The listing builds one solid part. Answer for the finished solid, in the listing's coordinates (mm). Round coordinates to 2 decimals unless told otherwise and drop trailing zeros. Write each loop counter-clockwise with the first axis right and the second up, starting at its lowest first coordinate (ties: lowest second). Pieces come first, ordered by that corner, then holes. Notation, with made-up numbers: M 16,-7.5 L 26,-7.5 A25 ccw 26,7.5 Z; hole C 36.5,72.5 d11. An arc over 180 degrees is marked long. Answer as CSV lines item,"result". Start each with the question number.
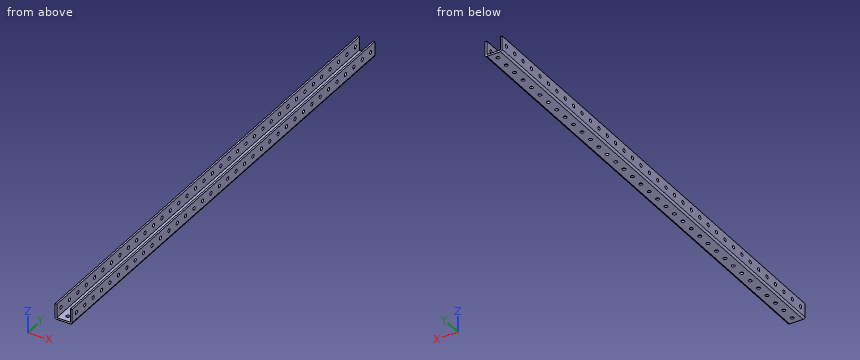
from build123d import *

# Parameters (mm, degrees)
F1_DEPTH = 914.4
F2_R     = 3.175
F3_DEPTH = 28.576
F4_R     = 3.175
F5_DEPTH = 31.751


with BuildPart() as f1:
    # F0 (on Front) → F1 (new body)
    with BuildSketch(Plane.XZ):
        with BuildLine():
            Line((-12.7, -14.2875), (12.7, -14.2875))
            ThreePointArc((12.7, -14.2875), (14.945064, -13.357564), (15.875, -11.1125))
            Line((15.875, -11.1125), (15.875, 14.2875))
            Line((15.875, 14.2875), (12.7, 14.2875))
            Line((12.7, 14.2875), (12.7, -11.1125))
            Line((12.7, -11.1125), (-12.7, -11.1125))
            Line((-12.7, -11.1125), (-12.7, 14.2875))
            Line((-12.7, 14.2875), (-15.875, 14.2875))
            Line((-15.875, 14.2875), (-15.875, -11.1125))
            ThreePointArc((-15.875, -11.1125), (-14.945064, -13.357564), (-12.7, -14.2875))
        make_face()
    extrude(amount=F1_DEPTH)

    # F2 (on face) → F3 (cut, through all)
    with BuildSketch(Plane(origin=(0, 0, -14.2875), x_dir=(1, 0, 0), z_dir=(0, 0, -1))):
        with Locations((0, 12.7)):
            Circle(F2_R)
        with Locations((0, 38.1)):
            Circle(F2_R)
        with Locations((0, 63.5)):
            Circle(F2_R)
        with Locations((0, 88.9)):
            Circle(F2_R)
        with Locations((0, 114.3)):
            Circle(F2_R)
        with Locations((0, 139.7)):
            Circle(F2_R)
        with Locations((0, 165.1)):
            Circle(F2_R)
        with Locations((0, 190.5)):
            Circle(F2_R)
        with Locations((0, 215.9)):
            Circle(F2_R)
        with Locations((0, 241.3)):
            Circle(F2_R)
        with Locations((0, 266.7)):
            Circle(F2_R)
        with Locations((0, 292.1)):
            Circle(F2_R)
        with Locations((0, 317.5)):
            Circle(F2_R)
        with Locations((0, 342.9)):
            Circle(F2_R)
        with Locations((0, 368.3)):
            Circle(F2_R)
        with Locations((0, 393.7)):
            Circle(F2_R)
        with Locations((0, 419.1)):
            Circle(F2_R)
        with Locations((0, 444.5)):
            Circle(F2_R)
        with Locations((0, 469.9)):
            Circle(F2_R)
        with Locations((0, 495.3)):
            Circle(F2_R)
        with Locations((0, 520.7)):
            Circle(F2_R)
        with Locations((0, 546.1)):
            Circle(F2_R)
        with Locations((0, 571.5)):
            Circle(F2_R)
        with Locations((0, 596.9)):
            Circle(F2_R)
        with Locations((0, 622.3)):
            Circle(F2_R)
        with Locations((0, 647.7)):
            Circle(F2_R)
        with Locations((0, 673.1)):
            Circle(F2_R)
        with Locations((0, 698.5)):
            Circle(F2_R)
        with Locations((0, 723.9)):
            Circle(F2_R)
        with Locations((0, 749.3)):
            Circle(F2_R)
        with Locations((0, 774.7)):
            Circle(F2_R)
        with Locations((0, 800.1)):
            Circle(F2_R)
        with Locations((0, 825.5)):
            Circle(F2_R)
        with Locations((0, 850.9)):
            Circle(F2_R)
        with Locations((0, 876.3)):
            Circle(F2_R)
        with Locations((0, 901.7)):
            Circle(F2_R)
    extrude(amount=-F3_DEPTH, mode=Mode.SUBTRACT)

    # F4 (on face) → F5 (cut, through all)
    with BuildSketch(Plane(origin=(-15.875, 0, 0), x_dir=(0, -1, 0), z_dir=(-1, 0, 0))):
        with Locations((12.700011, 1.5875)):
            Circle(F4_R)
        with Locations((38.100011, 1.5875)):
            Circle(F4_R)
        with Locations((63.500011, 1.5875)):
            Circle(F4_R)
        with Locations((88.900011, 1.5875)):
            Circle(F4_R)
        with Locations((114.300011, 1.5875)):
            Circle(F4_R)
        with Locations((139.700011, 1.5875)):
            Circle(F4_R)
        with Locations((165.100011, 1.5875)):
            Circle(F4_R)
        with Locations((190.500011, 1.5875)):
            Circle(F4_R)
        with Locations((215.900011, 1.5875)):
            Circle(F4_R)
        with Locations((241.300011, 1.5875)):
            Circle(F4_R)
        with Locations((266.700011, 1.5875)):
            Circle(F4_R)
        with Locations((292.100011, 1.5875)):
            Circle(F4_R)
        with Locations((317.500011, 1.5875)):
            Circle(F4_R)
        with Locations((342.900011, 1.5875)):
            Circle(F4_R)
        with Locations((368.300011, 1.5875)):
            Circle(F4_R)
        with Locations((393.700011, 1.5875)):
            Circle(F4_R)
        with Locations((419.100011, 1.5875)):
            Circle(F4_R)
        with Locations((444.500011, 1.5875)):
            Circle(F4_R)
        with Locations((469.900011, 1.5875)):
            Circle(F4_R)
        with Locations((495.300011, 1.5875)):
            Circle(F4_R)
        with Locations((520.700011, 1.5875)):
            Circle(F4_R)
        with Locations((546.100011, 1.5875)):
            Circle(F4_R)
        with Locations((571.500011, 1.5875)):
            Circle(F4_R)
        with Locations((596.900011, 1.5875)):
            Circle(F4_R)
        with Locations((622.300011, 1.5875)):
            Circle(F4_R)
        with Locations((647.700011, 1.5875)):
            Circle(F4_R)
        with Locations((673.100011, 1.5875)):
            Circle(F4_R)
        with Locations((698.500011, 1.5875)):
            Circle(F4_R)
        with Locations((723.900011, 1.5875)):
            Circle(F4_R)
        with Locations((749.300011, 1.5875)):
            Circle(F4_R)
        with Locations((774.700011, 1.5875)):
            Circle(F4_R)
        with Locations((800.100011, 1.5875)):
            Circle(F4_R)
        with Locations((825.500011, 1.5875)):
            Circle(F4_R)
        with Locations((850.900011, 1.5875)):
            Circle(F4_R)
        with Locations((876.300011, 1.5875)):
            Circle(F4_R)
        with Locations((901.700011, 1.5875)):
            Circle(F4_R)
    extrude(amount=-F5_DEPTH, mode=Mode.SUBTRACT)


solid = f1.part
Q1. Each of these flat-tipped pins is pushed along its axis until it touches: P1, Ø5.5, axis at y = -114.3, z = 1.59, coming from the -X side; P2, Ø10, axis at x = 0.5, y = -714.5, coming from the +Z side. Where does it stop, or does it pass through?
Q2. Straight lines are drawn through the part: L1, parallel to X at y = -342.9, z = -12.05 (3 decimals); L2, parallel to X at y = -570, z = -5 (3 decimals); L3, parallel to Z at x = 9, y = -224. For each, find the intervals that lie inside material, in ascending order.
Q3. Find section A-A (z = 9.25). Determine the outline of the cut face in (x, y) (3 decimals).
Reported:
1,P1,"passes through"
1,P2,"stops at z = -11.11"
2,L1,"x = -15.733 to -3.175, 3.175 to 15.733"
2,L2,"x = -15.875 to -12.7, 12.7 to 15.875"
2,L3,"z = -14.29 to -11.11"
3,outline,"M -15.875,-914.4 L -12.7,-914.4 L -12.7,0 L -15.875,0 Z; M 12.7,-914.4 L 15.875,-914.4 L 15.875,0 L 12.7,0 Z"
